Read the model definition and answer for the solid it produces. Units are mm, in the model's axes. Coordinates: 2 decimals unless noted, no trailing zeros. Loops run counter-clockwise (first coordinate to the right, second up) from the corner with the lowest first, then second, coordinate; pieces in that order, holes last. Notation, with made-up numbers: (39.5, -27) -> (79.5, -27) arc R11 cw to (79.5, -8) -> close; hole circle Ø9 at (2, 83). An arc over 180 degrees is marked (long way). Answer as a JSON object with one key per item and string values. Group by question number.
1) Section B-B, the plane z = 2.25 is taken. Count the separate pieces of the cut face and the enclosed holes in it, plus the area to 3 significant figures.
2) Consider probe 1 along X at (y, z) = (-75.5, 5.25); probe 2 along X at (y, z) = (-43, 3.5); probe 3 along Y at (x, z) = (212, 3.75). Determine where each line is inside the solid, lowest interval first. Write a range as [from, to].
3) Section A-A, the plane x = 85.5 is taken. Give the vertices of the cut face in (y, z), plus the area to 3 significant figures.
4) Flat-ended cylindrical pins translate along their axes: P1, Ø1.9, axis at x = 247.5, z = 2.5, coming from the -Y side; P2, Ø1.9, axis at x = 247.5, z = 2.5, coming from the +Y side. Find the tip coordinate at first contact, or state that the pin passes through.
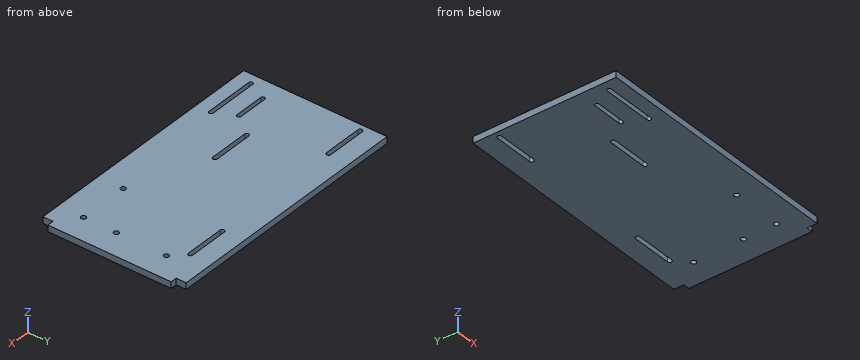
from build123d import *

# Parameters (mm, degrees)
SKETCH3_R           = 2.5
BOSS_EXTRUDE1_DEPTH = 6.35


with BuildPart() as part:
    # Sketch3 → Boss-Extrude1 (new body)
    with BuildSketch(Plane.XY):
        Polygon((244.584917863, 41.962665812), (-7.908318612, 41.962665812), (-7.908318612, -101.354312852), (244.584917863, -101.354312852), (244.584917863, -91.354312852), (250.934917863, -91.354312852), (250.934917863, 31.962665812), (244.584917863, 31.962665812), align=None)
        with Locations((225.534917863, -43.037334188)):
            Circle(SKETCH3_R, mode=Mode.SUBTRACT)
        with Locations((225.534917863, 6.962665812)):
            Circle(SKETCH3_R, mode=Mode.SUBTRACT)
        with Locations((225.534917863, -75.954312852)):
            Circle(SKETCH3_R, mode=Mode.SUBTRACT)
        with Locations((175.534917863, -75.954312852)):
            Circle(SKETCH3_R, mode=Mode.SUBTRACT)
        with BuildLine():
            Line((58.748599203, -43.204312852), (98.748599203, -43.204312852))
            ThreePointArc((98.748599203, -43.204312852), (100.898599203, -45.354312852), (98.748599203, -47.504312852))
            Line((98.748599203, -47.504312852), (58.748599203, -47.504312852))
            ThreePointArc((58.748599203, -47.504312852), (56.598599203, -45.354312852), (58.748599203, -43.204312852))
        make_face(mode=Mode.SUBTRACT)
        with BuildLine():
            Line((-1.261400797, 22.685687148), (38.738599203, 22.685687148))
            ThreePointArc((38.738599203, 22.685687148), (40.888599203, 20.535687148), (38.738599203, 18.385687148))
            Line((38.738599203, 18.385687148), (-1.261400797, 18.385687148))
            ThreePointArc((-1.261400797, 18.385687148), (-3.411400797, 20.535687148), (-1.261400797, 22.685687148))
        make_face(mode=Mode.SUBTRACT)
        with BuildLine():
            Line((172.288599203, 22.685687148), (212.288599203, 22.685687148))
            ThreePointArc((212.288599203, 22.685687148), (214.438599203, 20.535687148), (212.288599203, 18.385687148))
            Line((212.288599203, 18.385687148), (172.288599203, 18.385687148))
            ThreePointArc((172.288599203, 18.385687148), (170.138599203, 20.535687148), (172.288599203, 22.685687148))
        make_face(mode=Mode.SUBTRACT)
        with BuildLine():
            Line((12.091681388, -64.354312852), (42.091681388, -64.354312852))
            ThreePointArc((42.091681388, -64.354312852), (44.091681388, -66.354312852), (42.091681388, -68.354312852))
            Line((42.091681388, -68.354312852), (12.091681388, -68.354312852))
            ThreePointArc((12.091681388, -68.354312852), (10.091681388, -66.354312852), (12.091681388, -64.354312852))
        make_face(mode=Mode.SUBTRACT)
        with BuildLine():
            Line((2.091681388, -84.354312852), (52.091681388, -84.354312852))
            ThreePointArc((52.091681388, -84.354312852), (54.091681388, -86.354312852), (52.091681388, -88.354312852))
            Line((52.091681388, -88.354312852), (2.091681388, -88.354312852))
            ThreePointArc((2.091681388, -88.354312852), (0.091681388, -86.354312852), (2.091681388, -84.354312852))
        make_face(mode=Mode.SUBTRACT)
    extrude(amount=BOSS_EXTRUDE1_DEPTH)


solid = part.part
Determined:
{
 "1": {"separate pieces": "1", "enclosed holes": "9", "area": "36,000 mm²"},
 "2": {"probe 1": "[-7.91, 173.08], [177.99, 223.08], [227.99, 250.93]", "probe 2": "[-7.91, 223.04], [228.03, 250.93]", "probe 3": "[-101.35, 18.39], [22.69, 41.96]"},
 "3": {"outline": "(-101.35, 0) -> (-47.5, 0) -> (-47.5, 6.35) -> (-101.35, 6.35) -> close; (-43.2, 0) -> (41.96, 0) -> (41.96, 6.35) -> (-43.2, 6.35) -> close", "area": "883 mm²"},
 "4": {"P1": "y = -91.35", "P2": "y = 31.96"}
}
